from build123d import *

# Parameters (mm, degrees)
SKETCH2_R           = 30
BOSS_EXTRUDE1_DEPTH = 42
SKETCH2_4_R         = 38.5
BOSS_EXTRUDE2_DEPTH = 15
SKETCH3_R           = 3
CUT_EXTRUDE1_DEPTH  = 10
SKETCH4_R           = 3
CUT_EXTRUDE2_DEPTH  = 10


with BuildPart() as part:
    # Sketch2 → Boss-Extrude1 (new body)
    with BuildSketch(Plane.XY):
        Circle(SKETCH2_R)
    extrude(amount=BOSS_EXTRUDE1_DEPTH)

    # Sketch2_4 → Boss-Extrude2 (add)
    with BuildSketch(Plane.XY):
        Circle(SKETCH2_4_R)
    extrude(amount=-BOSS_EXTRUDE2_DEPTH)

    # Sketch3 → Cut-Extrude1 (cut)
    with BuildSketch(Plane(origin=(0, 0, -15), x_dir=(-1, 0, 0), z_dir=(0, 0, -1))):
        with Locations((0, 25)):
            Circle(SKETCH3_R)
        with Locations((25, 0)):
            Circle(SKETCH3_R)
        with Locations((0, -25)):
            Circle(SKETCH3_R)
        with Locations((-25, 0)):
            Circle(SKETCH3_R)
    extrude(amount=-CUT_EXTRUDE1_DEPTH, mode=Mode.SUBTRACT)

    # Sketch4 → Cut-Extrude2 (cut)
    with BuildSketch(Plane.XY.offset(42)):
        with Locations((0, 25)):
            Circle(SKETCH4_R)
        with Locations((17.67766953, 17.67766953)):
            Circle(SKETCH4_R)
        with Locations((25, 0)):
            Circle(SKETCH4_R)
        with Locations((17.67766953, -17.67766953)):
            Circle(SKETCH4_R)
        with Locations((0, -25)):
            Circle(SKETCH4_R)
        with Locations((-17.67766953, -17.67766953)):
            Circle(SKETCH4_R)
        with Locations((-25, 0)):
            Circle(SKETCH4_R)
        with Locations((-17.67766953, 17.67766953)):
            Circle(SKETCH4_R)
    extrude(amount=-CUT_EXTRUDE2_DEPTH, mode=Mode.SUBTRACT)


solid = part.part
Model file for the job. Use its own axes, mm. A direction names the side the tool comes from. Coordinates: 2 decimals unless noted, no trailing zeros. Order: outer loops, then holes, each group sorted by start corner. A loop starts at its lowest first (then second) coordinate and runs counter-clockwise, first axis right, second up. Notation, with made-up numbers: M 41,-0.5 L 74,-0.5 A10 cw 74,10.5 Z; hole C 60,1.5 d5. An arc over 180 degrees is marked long. Return JSON: item names as keys, results as strings.
1. Saw through at C-C (z = 19.5). Give the cut face in (x, y).
Ans:
{"outline": "C 0,0 d60"}
2. Flat gauge pins, fed straight in: pin 1 (3 mm diameter, centred on x = 17.5, y = -18, fed in from +Z); pin 2 (3 mm diameter, centred on x = 26, z = 3, fed in from +Y); pin 3 (4 mm diameter, centred on x = 1.5, z = 17, fed in from +Y). Where does each tip first touch, or does it go through?
Ans:
{"pin 1": "z = 32", "pin 2": "y = 17.31", "pin 3": "y = 30"}
3. Pull direction Y, two halves, no side cores. Call faces 4 (the face through (-25, 0, -5)), 5 (the face through (0, 0, 42)), 6 (the face through (-29.97, 1.32, 20.71)): +Y half, -Y half, draft (parallel to the pull), parting line (faces both ways), or undercut.
Ans:
{"face 4": "undercut", "face 5": "draft", "face 6": "parting line"}
4. Saw through at B-B (x = -25). Give the cut face in (y, z), and give its area (3 significant figures).
Ans:
{"outline": "M -29.28,-15 L -3,-15 L -3,-5 L 3,-5 L 3,-15 L 29.28,-15 L 29.28,0 L 16.58,0 L 16.58,42 L 3,42 L 3,32 L -3,32 L -3,42 L -16.58,42 L -16.58,0 L -29.28,0 Z", "area": "2,150 mm^2"}
5. Drill centre lines: probe 1 along Y at (x, z) = (0, 38.75); probe 2 along X at (y, z) = (19.5, 34); probe 3 along Y at (x, z) = (15.5, 38). Where is each one in solid material? Low to high.
Ans:
{"probe 1": "-30 to -28, -22 to 22, 28 to 30", "probe 2": "-22.8 to -20.06, -15.29 to 15.29, 20.06 to 22.8", "probe 3": "-25.69 to -19.74, -15.61 to 15.61, 19.74 to 25.69"}
6. Tool access for faces 1 (the face through (0, 25, -5)), 2 (the face through (17.03, 14.75, 37.07)), 3 (the face through (-30.55, -23.43, -7.4)): list every direction of +Z, -Z, +X, -X, +Y, -Y with a clear straight run to the whole face (end or side of a thin tool).
Ans:
{"face 1": "-Z", "face 2": "+Z", "face 3": "+Z, -Z"}
7. Saw through at A-A (y = 0). Give the cut face in (x, z), and give its area (4 significant figures).
Ans:
{"outline": "M -38.5,-15 L -28,-15 L -28,-5 L -22,-5 L -22,-15 L 22,-15 L 22,-5 L 28,-5 L 28,-15 L 38.5,-15 L 38.5,0 L 30,0 L 30,42 L 28,42 L 28,32 L 22,32 L 22,42 L -22,42 L -22,32 L -28,32 L -28,42 L -30,42 L -30,0 L -38.5,0 Z", "area": "3,435 mm^2"}
